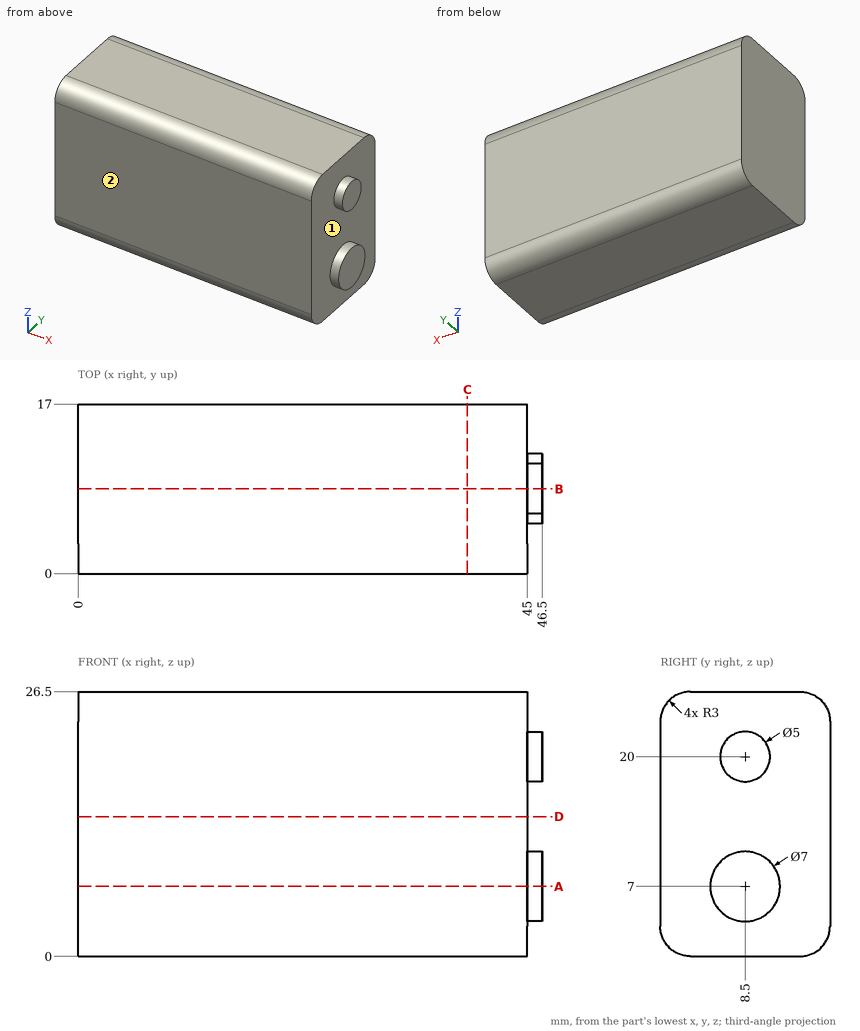
Print and shaded views of the part. All mm, measured from the part's lowest x, y and z. A direction names the side the tool comes from. Round coordinates to 2 decimals unless told otherwise and drop trailing zeros. Write each loop counter-clockwise with the first axis right and the second up, starting at its lowest first coordinate (ties: lowest second). Pieces come first, ordered by that corner, then holes. Notation, with made-up numbers: (78.25, 83) -> (124.25, 83) arc R23 ccw to (124.25, 93) -> close; hole circle Ø4 at (-19, 62). An arc over 180 degrees is marked (long way). Write item = value, one per line.
(1) Band-saw the part on B-B (y = 8.5). Give the cut face in (x, z).
Answer:
outline = (0, 0) -> (45, 0) -> (45, 3.5) -> (46.5, 3.5) -> (46.5, 10.5) -> (45, 10.5) -> (45, 17.5) -> (46.5, 17.5) -> (46.5, 22.5) -> (45, 22.5) -> (45, 26.5) -> (0, 26.5) -> close
(2) Band-saw the part on A-A (z = 7). Give the cut face in (x, y).
Answer:
outline = (0, 0) -> (45, 0) -> (45, 5) -> (46.5, 5) -> (46.5, 12) -> (45, 12) -> (45, 17) -> (0, 17) -> close
(3) Flat gauge pins, fed straight in: pin 1 (6 mm diameter, centred on y = 11, z = 19.5, fed in from +X); pin 2 (3 mm diameter, centred on y = 10.5, z = 23.5, fed in from +X). Where does each tip first touch, or does it go through?
Answer:
pin_1 = 46.5
pin_2 = 45
(4) Tool access for the marked faces 1 and 2: list every direction of +Z, -Z, +X, -X, +Y, -Y with a clear straight run to the whole face (end or side of a thin tool).
Answer:
face_1 = +X
face_2 = +Z, -Z, +X, -X, -Y
(5) Band-saw the part on C-C (x = 39). Give the cut face in (y, z).
Answer:
outline = (0, 3) arc R3 ccw to (3, 0) -> (14, 0) arc R3 ccw to (17, 3) -> (17, 23.5) arc R3 ccw to (14, 26.5) -> (3, 26.5) arc R3 ccw to (0, 23.5) -> close
(6) Band-saw the part on D-D (z = 14). Give the cut face in (x, y), then the cut area to 3 significant figures.
Answer:
outline = (0, 0) -> (45, 0) -> (45, 17) -> (0, 17) -> close
area = 765 mm2
(7) Probe L1, parallel to X at y = 1, z = 4.5; L2, parallel to Z at x = 5, y = 15; L3, parallel to Z at x = 4, y = 15.25. List the from-to ranges inside material, lowest first.
Answer:
L1 = 0 to 45
L2 = 0.17 to 26.33
L3 = 0.27 to 26.23
